```python
from build123d import *

# Parameters (mm, degrees)
F0_W     = 52
F0_H     = 60
F0_R     = 2.5
F1_DEPTH = 3
F2_W     = 52
F2_H     = 42
F3_DEPTH = 13
F4_SIZE  = 3
F5_SIZE  = 3
F6_SIZE  = 1
F7_SIZE  = 1


with BuildPart() as f1:
    # F0 (on Top) → F1 (new body)
    with BuildSketch(Plane.XY):
        Rectangle(F0_W, F0_H)
        with Locations((-22, -26)):
            Circle(F0_R, mode=Mode.SUBTRACT)
        with Locations((22, -26)):
            Circle(F0_R, mode=Mode.SUBTRACT)
        with Locations((-22, 26)):
            Circle(F0_R, mode=Mode.SUBTRACT)
        with Locations((22, 26)):
            Circle(F0_R, mode=Mode.SUBTRACT)
    extrude(amount=F1_DEPTH)

    # F2 (on face) → F3 (join)
    with BuildSketch(Plane.XY.offset(3)):
        with Locations((0, 1)):
            Rectangle(F2_W, F2_H)
    extrude(amount=F3_DEPTH)

    # F4
    f4_edges = [f1.edges().sort_by_distance(p)[0] for p in [
        (0, -20, 16),
    ]]
    chamfer(f4_edges, length=F4_SIZE)

    # F5
    f5_edges = [f1.edges().sort_by_distance(p)[0] for p in [
        (0, 22, 16),
    ]]
    chamfer(f5_edges, length=F5_SIZE)

    # F6
    f6_edges = [f1.edges().sort_by_distance(p)[0] for p in [
        (-26, 1, 16),
    ]]
    chamfer(f6_edges, length=F6_SIZE)

    # F7
    f7_edges = [f1.edges().sort_by_distance(p)[0] for p in [
        (26, 1, 16),
    ]]
    chamfer(f7_edges, length=F7_SIZE)


solid = f1.part
```
The listing builds one solid part. Answer for the finished solid, in the listing's coordinates (mm). A direction names the side the tool comes from. Give positions to 0.01 mm unless a question says otherwise; leave off trailing zeros. Order: outer loops, then holes, each group sorted by start corner. A loop starts at its lowest first (then second) coordinate and runs counter-clockwise, first axis right, second up. Notation, with made-up numbers: M 47,28.25 L 102,28.25 A18 ccw 102,37.25 Z; hole C 19.25,-15 d8. An arc over 180 degrees is marked long. Put each result on its own line as item: value. Start each with the question number.
Item 1: The part is cut by section A-A, the plane x = -22. Determine the outline of the cut face in (y, z).
Item 2: The part is cut by section D-D, the plane x = -10. Determine the outline of the cut face in (y, z).
Item 3: The part is cut by section C-C, the plane y = 26. Determine the outline of the cut face in (x, z), and give its area (3 significant figures).
Item 4: For a pull along X with two mould halves and no side action, classify faces 1 (the face through (-23.84, 27.69, 1.48)), 2 (the face through (-26, 0, 7)), 3 (the face through (26, 0, 7)) as +X half, -X half, draft (parallel to the pull), parting line (faces both ways), or undercut.
Item 5: The part is cut by section B-B, the plane z = 2.25. Determine the outline of the cut face in (x, y), and give its area (3 significant figures).
Item 6: Find the intervals of material crossed by line 1 along Y through (x, z) = (-22, 1.4); line 2 along Z through (x, y) = (-16.5, 20); line 3 along Z through (x, y) = (-0.5, 24), in increasing order.
Item 7: Which of the six approach directions +Z, -Z, +X, -X, +Y, -Y give full straight-line access (tool end or side, diameter ignored) to faces 4 (the face through (0, -25, 3)), 5 (the face through (0, 1, 16)), 6 (the face through (0, 26, 3))?
Item 8: Flat-ended cylindrical pins translate along their axes: P1, Ø1, axis at x = 11.5, y = 10.5, coming from the -Z side; P2, Ø8, axis at x = -10.5, z = 14, coming from the +Y side; P3, Ø9, axis at x = 10.5, y = 27, coming from the +Z side; P4, Ø4, axis at x = -6, y = 22, coming from the +Z side. Find the tip coordinate at first contact, or state that the pin passes through.
Answer key:
1. outline: M -30,0 L -28.5,0 L -28.5,3 L -30,3 Z; M -23.5,0 L 23.5,0 L 23.5,3 L 22,3 L 22,13 L 19,16 L -17,16 L -20,13 L -20,3 L -23.5,3 Z; M 28.5,0 L 30,0 L 30,3 L 28.5,3 Z
2. outline: M -30,0 L 30,0 L 30,3 L 22,3 L 22,13 L 19,16 L -17,16 L -20,13 L -20,3 L -30,3 Z
3. outline: M -26,0 L -24.5,0 L -24.5,3 L -26,3 Z; M -19.5,0 L 19.5,0 L 19.5,3 L -19.5,3 Z; M 24.5,0 L 26,0 L 26,3 L 24.5,3 Z
3. area: 126 mm²
4. face 1: undercut
4. face 2: -X half
4. face 3: +X half
5. outline: M -26,-30 L 26,-30 L 26,30 L -26,30 Z; hole C -22,-26 d5; hole C -22,26 d5; hole C 22,-26 d5; hole C 22,26 d5
5. area: 3,040 mm²
6. line 1: y = -30 to -28.5, -23.5 to 23.5, 28.5 to 30
6. line 2: z = 0 to 15
6. line 3: z = 0 to 3
7. face 4: +Z, +X, -X, -Y
7. face 5: +Z, +X, -X, +Y, -Y
7. face 6: +Z, +X, -X, +Y
8. P1: stops at z = 0
8. P2: stops at y = 22
8. P3: stops at z = 3
8. P4: stops at z = 15
